from build123d import *

# Parameters (mm, degrees)
SKETCH_1_R          = 10
EXTRUDE_1_DEPTH     = 50
SKETCH_2_R          = 11
EXTRUDE_2_DEPTH     = 10
CHAMFER_1_SIZE      = 4
CHAMFER_1_SIZE2     = 1.07179677
SKETCH_3_R          = 10
SKETCH_3_R_2        = 9
CUT_EXTRUDE_1_DEPTH = 1


with BuildPart() as part:
    # Эскиз1 → Бобышка-Вытянуть1 (new body)
    with BuildSketch(Plane(origin=(0, 0, 0), x_dir=(1, 0, 0), z_dir=(0, 1, 0))):
        with Locations(Location((0, 0, 0), (0, 0, 270))):
            Circle(SKETCH_1_R)
    extrude(amount=EXTRUDE_1_DEPTH)

    # Эскиз2 → Бобышка-Вытянуть2 (add)
    with BuildSketch(Plane.XZ):
        with Locations(Location((0, 0, 0), (0, 0, 270))):
            Circle(SKETCH_2_R)
    extrude(amount=EXTRUDE_2_DEPTH)

    # Фаска1
    chamfer_1_edges = [part.edges().sort_by_distance(p)[0] for p in [
        (0, 50, -10),
    ]]
    chamfer_1_side = [part.faces().sort_by_distance(p)[0] for p in [
        (0, 25, -10),
    ]]
    chamfer(chamfer_1_edges, length=CHAMFER_1_SIZE, length2=CHAMFER_1_SIZE2, reference=chamfer_1_side[0])

    # Эскиз3 → Вырез-Вытянуть1 (cut)
    with BuildSketch(Plane(origin=(0, 0, 0), x_dir=(1, 0, 0), z_dir=(0, 1, 0))):
        with Locations(Location((0, 0, 0), (0, 0, 270))):
            Circle(SKETCH_3_R)
        with Locations(Location((0, 0, 0), (0, 0, 270))):
            Circle(SKETCH_3_R_2, mode=Mode.SUBTRACT)
    extrude(amount=CUT_EXTRUDE_1_DEPTH, mode=Mode.SUBTRACT)


solid = part.part
Verification items for the finished model (mm, model axes). A direction names the side the tool comes from. Coordinates: 2 decimals unless noted, no trailing zeros. Order: outer loops, then holes, each group sorted by start corner. A loop starts at its lowest first (then second) coordinate and runs counter-clockwise, first axis right, second up. Notation, with made-up numbers: M 29,37.25 L 68,37.25 A4 ccw 68,41.25 Z; hole C 76,46 d8. An arc over 180 degrees is marked long. One line per item, written item: value. Start each with the question number.
Item 1: Sectioned sample at A-A on z = 0. Record the cut outline in (x, y), then the cut area to 3 significant figures.
Item 2: Access from +Z, -Z, +X, -X, +Y, -Y to the whole of each face (thin tool, end or side, straight path). Record for faces 4 (the cylindrical face through (-10.74, -4.93, 2.38)), 5 (the flat face through (-9, 0, -2)).
Item 3: Depth check by flat-ended pin: P1, Ø5, axis at y = 8, z = -5, coming from the +X side; P2, Ø10, axis at y = 37, z = 7, coming from the +X side; P3, Ø12, axis at y = 27.5, z = -0.5, coming from the +X side. Enter the tip coordinate at first touch or a pass-through.
Item 4: Thickness scan on probe 1 along X at (y, z) = (28.5, -0.5); probe 2 along Y at (x, z) = (-10, -2.25); probe 3 along Z at (x, y) = (3.25, 44). Record the ranges inside material, lowest first.
Item 5: Sectioned sample at B-B on x = 0. Record the cut outline in (y, z).
Item 6: Mould release check, pull along Y, two halves, no side actions. Record for faces 1 (the cylindrical face through (2.703, 0.493, 8.584)), 2 (the flat face through (0, 50, 0)), 3 (the cylindrical face through (-9.76, 23.18, -2.17)): pulls with the +Y half, pulls with the -Y half, needs draft (parallel to the pull), parting line crosses it, or undercut.
Item 7: Sectioned sample at C-C on y = -1. Record the cut outline in (x, z).
Calculated:
1. outline: M -11,-10 L 11,-10 L 11,0 L 9,0 L 9,1 L 10,1 L 10,46 L 8.93,50 L -8.93,50 L -10,46 L -10,1 L -9,1 L -9,0 L -11,0 Z
1. area: 1,210 mm^2
2. face 4: +Y, -Y
2. face 5: none
3. P1: x = 9.68
3. P2: x = 9.8
3. P3: x = 10
4. probe 1: -9.99 to 9.99
4. probe 2: -10 to 0
4. probe 3: -9.46 to 9.46
5. outline: M -10,-11 L 0,-11 L 0,-9 L 1,-9 L 1,-10 L 46,-10 L 50,-8.93 L 50,8.93 L 46,10 L 1,10 L 1,9 L 0,9 L 0,11 L -10,11 Z
6. face 1: undercut
6. face 2: pulls with the +Y half
6. face 3: needs draft
7. outline: C 0,0 d22
